Geometry: final body of the model. Coordinates: model frame, mm. A direction names the side the tool comes from. Give positions to 0.01 mm unless a question says otherwise; leave off trailing zeros. Write each loop counter-clockwise with the first axis right and the second up, starting at its lowest first coordinate (ties: lowest second). Pieces come first, ordered by that corner, then holes. Notation, with made-up numbers: (-35, 6) - (-7, 6) arc R18 cw to (-7, 21) - close; hole circle Ø11 at (10.5, 75.5). An arc over 180 degrees is marked (long way). Use CSV: the item, a comma, the result in double quotes. Start each with the question number.
(1) First-contact query: pin 1 Ø8 at (y, z) = (7, 10.5) entering from -X; pin 2 Ø6 at (x, z) = (-23, 1.5) entering from -Y; pin 3 Ø1.4 at (y, z) = (0.5, 4.5) entering from +X; pin 4 Ø5 at (x, z) = (-50, 11) entering from +Y. Flat tips, straight axial feed; report the tip coordinate or a pass-through.
(2) Line query: probe 1 along Z at (x, y) = (-93, 5.75); probe 2 along Y at (x, z) = (-55, 7); probe 3 along X at (y, z) = (8.75, 5.5). Output: solid intervals per line, ascending. Write a range as [from, to].
(3) Section A-A on x = -54.5. Output: boundary loops of the cut face in (y, z).
(4) Section C-C on x = 9.5. Output: boundary loops of the cut face in (y, z), and give its area (3 significant figures).
(5) Section B-B on z = 4. Output: boundary loops of the cut face in (x, y).
(6) Reachability of faces 1 (the flat face through (-66, 11, 0)), 2 (the flat face through (-66, 0, 9)), 3 (the flat face through (-66, 1, 9)) from +Z, -Z, +X, -X, +Y, -Y: full face, straight path, thin tool, end or side. Return the list, or none.
from build123d import *

# Parameters (mm, degrees)
SKETCH2_W                    = 130
SKETCH2_H                    = 20
BASE_FLANGE1_DEPTH           = 1
EDGE_FLANGE1_STRIP_W         = 5.4732
EDGE_FLANGE1_STRIP_H         = 1
EDGE_FLANGE1_STRIP_CUT_DEPTH = 130
EDGE_FLANGE1_DEPTH           = 130
EDGE_FLANGE2_DEPTH           = 18.2634
FILLET1_R                    = 2


# Sheet-metal steps are written as plain solids
with BuildPart() as part:
    # Sketch2 → Base-Flange1 (new body)
    with BuildSketch(Plane.XY):
        with Locations((-65, 10)):
            Rectangle(SKETCH2_W, SKETCH2_H)
    extrude(amount=-BASE_FLANGE1_DEPTH)

    # Edge-Flange1 strip (across the edge) → Edge-Flange1 strip cut (cut)
    with BuildSketch(Plane.YZ.offset(-130)):
        with Locations((-1, -0.5)):
            Rectangle(EDGE_FLANGE1_STRIP_W, EDGE_FLANGE1_STRIP_H)
    extrude(amount=EDGE_FLANGE1_STRIP_CUT_DEPTH, mode=Mode.SUBTRACT)

    # Edge-Flange1 section (across the edge) → Edge-Flange1 (add)
    with BuildSketch(Plane.YZ.offset(-130)):
        with BuildLine():
            Line((0, 0.7366), (0, 17))
            Line((0, 17), (1, 17))
            Line((1, 17), (1, 0.7366))
            ThreePointArc((1, 0.7366), (1.215745145, 0.215745145), (1.7366, 0))
            Line((1.7366, 0), (1.7366, -1))
            ThreePointArc((1.7366, -1), (0.508638364, -0.491361636), (0, 0.7366))
        make_face()
    extrude(amount=EDGE_FLANGE1_DEPTH)

    # Edge-Flange2 section (across the edge) → Edge-Flange2 (add)
    with BuildSketch(Plane(origin=(0.30510971, 1.7366, 0), x_dir=(-0.7071067811865438, 0, 0.7071067811865512), z_dir=(0, 1, 0))):
        with BuildLine():
            Line((-1, 0.30510971), (-1, 29.585786438))
            Line((-1, 29.585786438), (0, 29.585786438))
            Line((0, 29.585786438), (0, 0.30510971))
            ThreePointArc((0, 0.30510971), (0.056070336, 0.023225094), (0.215745145, -0.215745145))
            Line((0.215745145, -0.215745145), (-0.491361636, -0.922851926))
            ThreePointArc((-0.491361636, -0.922851926), (-0.867809196, -0.359458339), (-1, 0.30510971))
        make_face()
    extrude(amount=EDGE_FLANGE2_DEPTH)

    # Fillet1
    fillet1_edges = [part.edges().sort_by_distance(p)[0] for p in [
        (-130, 0.5, 17),
        (0, 0.5, 17),
        (21.578973317, 1.7366, 20.566756826),
        (21.578973317, 20, 20.566756826),
        (-130, 20, -0.5),
    ]]
    fillet(fillet1_edges, radius=FILLET1_R)


solid = part.part
Check values:
1,pin 1,"stops at x = 6.81"
1,pin 2,"stops at y = 0"
1,pin 3,"stops at x = 0"
1,pin 4,"stops at y = 1"
2,probe 1,"z = [-1, 0]"
2,probe 2,"y = [0, 1]"
2,probe 3,"x = [5.81, 7.22]"
3,outline,"(0, 0.74) arc R1.74 ccw to (1.74, -1) - (20, -1) - (20, 0) - (1.74, 0) arc R0.74 cw to (1, 0.74) - (1, 17) - (0, 17) - close"
4,outline,"(1.74, 7.78) - (20, 7.78) - (20, 9.19) - (1.74, 9.19) - close"
4,area,"25.8 mm²"
5,outline,"(-130, 0) - (0, 0) - (0, 1) - (-130, 1) - close; (4.31, 1.74) - (5.72, 1.74) - (5.72, 20) - (4.31, 20) - close"
6,face 1,"+Z, -X, +Y"
6,face 2,"+Z, -Z, +X, -X, -Y"
6,face 3,"+Z, +X, -X, +Y"
